Part model, mm, in its own coordinate system. Face numbers are marked on the shaded views. A direction names the side the tool comes from. Coordinates: 2 decimals unless noted, no trailing zeros. Order: outer loops, then holes, each group sorted by start corner. A loop starts at its lowest first (then second) coordinate and runs counter-clockwise, first axis right, second up. Notation, with made-up numbers: M -11.75,75.5 L -1.75,75.5 A26 cw -1.75,89.5 Z; hole C 21.25,79 d7. An arc over 180 degrees is marked long. Answer in a Markdown table with one row per item. Add a question column.
from build123d import *

# Parameters (mm, degrees)
F0_R     = 2.65
F1_DEPTH = 4
F2_R     = 3.75
F3_DEPTH = 15
F5_DEPTH = 4
F6_SIZE  = 0.3


with BuildPart() as f1:
    # F0 (on Right) → F1 (new body)
    with BuildSketch(Plane.YZ):
        Circle(F0_R)
    extrude(amount=F1_DEPTH)

    # F2 (on face) → F3 (join)
    with BuildSketch(Plane.YZ.offset(4)):
        Circle(F2_R)
    extrude(amount=F3_DEPTH)

    # F4 (on face) → F5 (cut)
    with BuildSketch(Plane.YZ.offset(19)):
        Polygon((2, -1.154701), (2, 1.154701), (0, 2.309401), (-2, 1.154701), (-2, -1.154701), (0, -2.309401), align=None)
    extrude(amount=-F5_DEPTH, mode=Mode.SUBTRACT)

    # F6
    f6_edges = [f1.edges().sort_by_distance(p)[0] for p in [
        (19, -3.75, 0),
        (4, -3.75, 0),
    ]]
    chamfer(f6_edges, length=F6_SIZE)


solid = f1.part
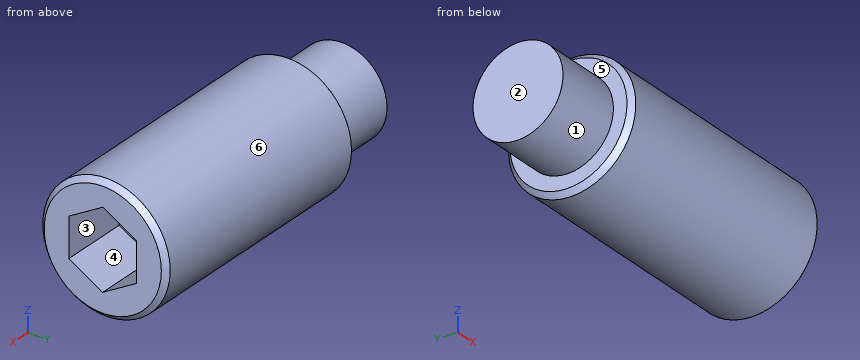
(1) Slice it at C-C (x = 3.5). List the corners of the cut face in (y, z), and give its area (3 significant figures).
(2) Wall check: line 1 (X direction, y = -0.75, z = 0.75); line 2 (X direction, y = 2.25, z = 2.5); line 3 (Y direction, x = 16.25, z = -0.25). Give the ranges that are in metal, low to high.
(3) Slice it at D-D (x = 8.5). List the corners of the cut face in (y, z).
(4) Pull direction Y, two halves, no side cores. Call the marked faces 1, 2, 3 and 4: pulls with the +Y half, pulls with the -Y half, needs draft (parallel to the pull), parting line crosses it, or undercut.
(5) Slice it at A-A (x = 16). List the corners of the cut face in (y, z).
(6) 3-axis set-ups, long thin cutter, end or side, ignore diameter. For the marked faces 5 and 6: which of +Z, -Z, +X, -X, +Y, -Y reach the whole face in a straight line?
(7) Drop a flat-ended pin along its axis: P1, Ø1, axis at x = 2.5, z = 1, coming from the -Y side. Give the stop position or say it passes through.
(8) Slice it at B-B (z = 0). List the corners of the cut face in (x, y), and give its area (3 significant figures).
Computed:
| question | item | result |
|---|---|---|
| 1 | outline | C 0,0 d5.3 |
| 1 | area | 22.1 mm^2 |
| 2 | line 1 | x = 0 to 15 |
| 2 | line 2 | x = 4 to 19 |
| 2 | line 3 | y = -3.74 to -2, 2 to 3.74 |
| 3 | outline | C 0,0 d7.5 |
| 4 | face 1 | parting line crosses it |
| 4 | face 2 | needs draft |
| 4 | face 3 | undercut |
| 4 | face 4 | undercut |
| 5 | outline | C 0,0 d7.5; hole M -2,-1.15 L 0,-2.31 L 2,-1.15 L 2,1.15 L 0,2.31 L -2,1.15 Z |
| 6 | face 5 | -X |
| 6 | face 6 | +X, -X |
| 7 | P1 | stops at y = -2.6 |
| 8 | outline | M 0,-2.65 L 4,-2.65 L 4,-3.45 L 4.3,-3.75 L 18.7,-3.75 L 19,-3.45 L 19,-2 L 15,-2 L 15,2 L 19,2 L 19,3.45 L 18.7,3.75 L 4.3,3.75 L 4,3.45 L 4,2.65 L 0,2.65 Z |
| 8 | area | 118 mm^2 |
